Job drawing, mm, ordinate dimensions from the low corner. One solid piece. A direction names the side the tool comes from. Round coordinates to 2 decimals unless told otherwise and drop trailing zeros. Loops run counter-clockwise (first coordinate to the right, second up) from the corner with the lowest first, then second, coordinate; pieces in that order, holes last.
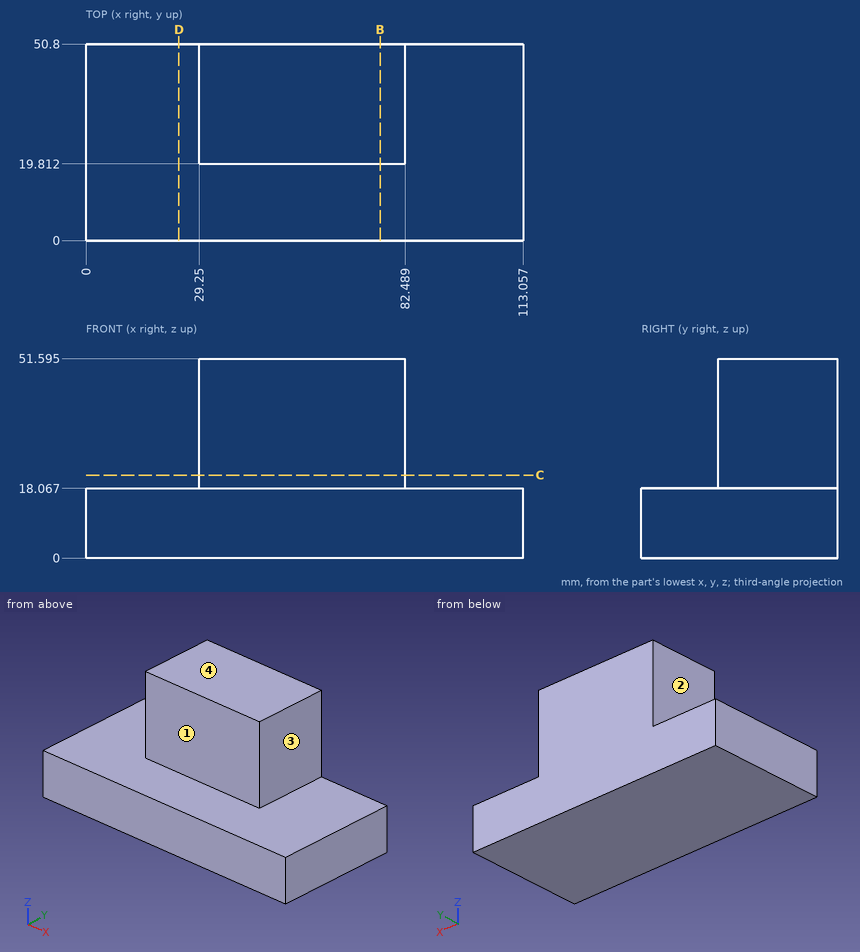
1) Slice it at D-D, the plane x = 24. Give the cut face in (y, z), then the cut area to 3 significant figures.
Values:
outline: (0, 0) - (50.8, 0) - (50.8, 18.07) - (0, 18.07) - close
area: 918 mm2
2) Slice it at B-B, the plane x = 76. Give the cut face in (y, z) (1 decimal), then the cut area to 3 significant figures.
Values:
outline: (0, 0) - (50.8, 0) - (50.8, 51.6) - (19.8, 51.6) - (19.8, 18.1) - (0, 18.1) - close
area: 1,960 mm2
3) Tool access for the marked faces 1, 2, 3 and 4: list every direction of +Z, -Z, +X, -X, +Y, -Y with a clear straight run to the whole face (end or side of a thin tool).
Values:
face 1: +Z, +X, -X, -Y
face 2: +Z, -X, +Y, -Y
face 3: +Z, +X, +Y, -Y
face 4: +Z, +X, -X, +Y, -Y
4) Slice it at C-C, the plane z = 21.5. Give the cut face in (x, y).
Values:
outline: (29.25, 19.81) - (82.49, 19.81) - (82.49, 50.8) - (29.25, 50.8) - close
5) Wall check: line 1 along Z through (x, y) = (99, 31.5); line 2 along X through (y, z) = (43, 28.5); line 3 along Y through (x, z) = (63.5, 24). Give the ranges that are in metal, low to high.
Values:
line 1: z = 0 to 18.07
line 2: x = 29.25 to 82.49
line 3: y = 19.81 to 50.8
6) Drop flat-ended pins along their axis: pin 1 Ø5 at (y, z) = (44, 40) entering from +X; pin 2 Ø10 at (x, z) = (61, 31.5) entering from -Y; pin 3 Ø15.5 at (y, z) = (38, 43) entering from -X. Give the stop position or say it passes through.
Values:
pin 1: stops at x = 82.49
pin 2: stops at y = 19.81
pin 3: stops at x = 29.25
